Build history of the part. All positions in model axes, mm. A direction names the side the tool comes from. Round coordinates to 2 decimals unless told otherwise and drop trailing zeros. Order: outer loops, then holes, each group sorted by start corner. A loop starts at its lowest first (then second) coordinate and runs counter-clockwise, first axis right, second up. Notation, with made-up numbers: M -29,-29 L 27,-29 A18 ccw 27,-25 Z; hole C 44.5,88 d5. An arc over 180 degrees is marked long. One line per question, with ' | ' between items. Start each with the question number.
Autodesk Inventor part; units mm, degrees
ref_plane "YZ Plane" through (0, 0, 0) normal (1, 0, 0) x (0, 1, 0)
ref_plane "XZ Plane" through (0, 0, 0) normal (0, 1, 0) x (-1, 0, 0)
ref_plane "XY Plane" through (0, 0, 0) normal (0, 0, 1) x (1, 0, 0)
sketch "Boceto1" plane through (0, 0, 0) normal (0, 0, 1) x (1, 0, 0)
  line L0 (75.85, 9) -> (75.85, -9)
  line L1 (75.85, 9) -> (95.85, 9)
  line L2 (95.85, -9) -> (95.85, 9)
  line L3 (105.85, -146.9) -> (105.85, 146.9)
  line L4 (105.85, 146.9) -> (112.15, 146.9)
  line L5 (112.15, 146.9) -> (112.15, 160)
  line L6 (112.15, 160) -> (105.85, 160)
  line L7 (105.85, 160) -> (105.85, 180)
  line L8 (105.85, 180) -> (-100.9, 180)
  line L9 (-100.9, 180) -> (-100.9, 160)
  line L10 (-100.9, 160) -> (-108.4, 160)
  line L11 (-108.4, 160) -> (-108.4, 145)
  line L12 (-108.4, 145) -> (-100.9, 145)
  line L13 (-100.9, 145) -> (-100.9, 142)
  line L14 (-100.9, 142) -> (-112.15, 142)
  line L15 (-112.15, 142) -> (-112.15, -142)
  line L16 (15.85, 9) -> (15.85, -9)
  line L17 (15.85, 9) -> (35.85, 9)
  line L18 (35.85, -9) -> (35.85, 9)
  line L19 (20.45, 169.8) -> (20.45, 163.3)
  line L20 (20.45, 163.3) -> (13.95, 163.3)
  line L21 (13.95, 163.3) -> (13.95, 169.8)
  line L22 (13.95, 169.8) -> (20.45, 169.8)
  line L23 (78.15, 169.8) -> (78.15, 163.3)
  line L24 (78.15, 163.3) -> (71.65, 163.3)
  line L25 (71.65, 163.3) -> (71.65, 169.8)
  line L26 (71.65, 169.8) -> (78.15, 169.8)
  line L27 (-4.15, 163.3) -> (-4.15, 169.8)
  line L28 (-4.15, 169.8) -> (2.35, 169.8)
  line L29 (2.35, 169.8) -> (2.35, 163.3)
  line L30 (2.35, 163.3) -> (-4.15, 163.3)
  line L31 (38.55, 169.8) -> (38.55, 163.3)
  line L32 (38.55, 163.3) -> (32.05, 163.3)
  line L33 (32.05, 163.3) -> (32.05, 169.8)
  line L34 (32.05, 169.8) -> (38.55, 169.8)
  line L35 (56.65, 169.8) -> (56.65, 163.3)
  line L36 (56.65, 163.3) -> (50.15, 163.3)
  line L37 (50.15, 163.3) -> (50.15, 169.8)
  line L38 (50.15, 169.8) -> (56.65, 169.8)
  line L39 (-14.65, 175.8) -> (-14.65, 157.7)
  line L40 (-14.65, 157.7) -> (-22.65, 157.7)
  line L41 (-22.65, 157.7) -> (-22.65, 175.8)
  line L42 (-22.65, 175.8) -> (-14.65, 175.8)
  line L43 (35.85, -9) -> (35.85, 9)
  line L44 (35.85, -9) -> (15.85, -9)
  line L45 (15.85, 9) -> (15.85, -9)
  line L46 (-112.15, 142) -> (-112.15, -142)
  line L47 (-112.15, -142) -> (-100.9, -142)
  line L48 (-100.9, -142) -> (-100.9, -145)
  line L49 (-100.9, -145) -> (-108.4, -145)
  line L50 (-108.4, -145) -> (-108.4, -160)
  line L51 (-108.4, -160) -> (-100.9, -160)
  line L52 (-100.9, -160) -> (-100.9, -180)
  line L53 (-100.9, -180) -> (105.85, -180)
  line L54 (105.85, -180) -> (105.85, -160)
  line L55 (105.85, -160) -> (112.15, -160)
  line L56 (112.15, -160) -> (112.15, -146.9)
  line L57 (112.15, -146.9) -> (105.85, -146.9)
  line L58 (105.85, -146.9) -> (105.85, 146.9)
  line L59 (95.85, -9) -> (95.85, 9)
  line L60 (95.85, -9) -> (75.85, -9)
  line L61 (75.85, 9) -> (75.85, -9)
  circle A0 centre (-103.8, -156.7) radius 1.5
  line L62 (-25.85, -52.4) -> (-25.85, -57.4)
  line L63 (-25.85, -57.4) -> (-8.15, -57.4)
  arc A1 (-3.15, -62.4) -> (-8.15, -57.4) centre (-8.15, -62.4) ccw
  line L64 (-3.15, -62.4) -> (-3.15, -87.4)
  line L65 (-3.15, -87.4) -> (-2.05, -87.4)
  line L66 (-2.05, -87.4) -> (-2.05, -107.4)
  line L67 (-2.05, -107.4) -> (-3.15, -107.4)
  line L68 (-3.15, -107.4) -> (-3.15, -169.7804)
  arc A2 (-8.15, -174.7804) -> (-3.15, -169.7804) centre (-8.15, -169.7804) ccw
  line L69 (-8.15, -174.7804) -> (-67.5256, -174.7804)
  line L70 (-67.5256, -174.7804) -> (-67.5256, -57.4)
  line L71 (-67.5256, -57.4) -> (-48.05, -57.4)
  line L72 (-48.05, -57.4) -> (-48.05, -52.4)
  line L73 (-48.05, -52.4) -> (-25.85, -52.4)
  line L74 (-112.15, 0) -> (-67.15, 0)
  line L75 (-67.15, 0) -> (-67.15, -40)
  line L76 (-67.15, -40) -> (-32.15, -40)
  line L77 (-32.15, -40) -> (-32.15, 40)
  line L78 (-32.15, 40) -> (-67.15, 40)
  line L79 (-67.15, 40) -> (-67.15, 0)
  line L80 (-37.15, 35) -> (-37.15, -35)
  line L81 (-37.15, -35) -> (-62.15, -35)
  line L82 (-62.15, -35) -> (-62.15, 0)
  line L83 (-62.15, 0) -> (-62.15, 35)
  line L84 (-62.15, 35) -> (-37.15, 35)
  circle A3 centre (-37.15, 35) radius 1.5
  circle A4 centre (-37.15, -35) radius 1.5
  circle A5 centre (-62.15, -35) radius 1.5
  circle A6 centre (-62.15, 35) radius 1.5
  circle A7 centre (-37.15, -35) radius 1.6
  circle A8 centre (-37.15, 35) radius 1.6
  circle A9 centre (-62.15, 35) radius 1.6
  circle A10 centre (-62.15, -35) radius 1.6
  line L85 (75.85, 9) -> (95.85, 9)
  line L86 (15.85, 9) -> (35.85, 9)
  line L87 (20.45, 169.8) -> (20.45, 163.3)
  line L88 (20.45, 163.3) -> (13.95, 163.3)
  line L89 (13.95, 163.3) -> (13.95, 169.8)
  line L90 (13.95, 169.8) -> (20.45, 169.8)
  line L91 (78.15, 169.8) -> (78.15, 163.3)
  line L92 (78.15, 163.3) -> (71.65, 163.3)
  line L93 (71.65, 163.3) -> (71.65, 169.8)
  line L94 (71.65, 169.8) -> (78.15, 169.8)
  line L95 (-4.15, 163.3) -> (-4.15, 169.8)
  line L96 (-4.15, 169.8) -> (2.35, 169.8)
  line L97 (2.35, 169.8) -> (2.35, 163.3)
  line L98 (2.35, 163.3) -> (-4.15, 163.3)
  line L99 (38.55, 169.8) -> (38.55, 163.3)
  line L100 (38.55, 163.3) -> (32.05, 163.3)
  line L101 (32.05, 163.3) -> (32.05, 169.8)
  line L102 (32.05, 169.8) -> (38.55, 169.8)
  line L103 (56.65, 169.8) -> (56.65, 163.3)
  line L104 (56.65, 163.3) -> (50.15, 163.3)
  line L105 (50.15, 163.3) -> (50.15, 169.8)
  line L106 (50.15, 169.8) -> (56.65, 169.8)
  line L107 (-14.65, 175.8) -> (-14.65, 157.7)
  line L108 (-14.65, 157.7) -> (-22.65, 157.7)
  line L109 (-22.65, 157.7) -> (-22.65, 175.8)
  line L110 (-22.65, 175.8) -> (-14.65, 175.8)
  line L111 (-100.9, 142) -> (-112.15, 142)
  line L112 (105.85, 146.9) -> (112.15, 146.9)
  line L113 (112.15, 146.9) -> (112.15, 160)
  line L114 (112.15, 160) -> (105.85, 160)
  line L115 (105.85, 160) -> (105.85, 180)
  line L116 (105.85, 180) -> (-100.9, 180)
  line L117 (-100.9, 180) -> (-100.9, 160)
  line L118 (-100.9, 160) -> (-108.4, 160)
  line L119 (-108.4, 160) -> (-108.4, 145)
  line L120 (-108.4, 145) -> (-100.9, 145)
  line L121 (-100.9, 145) -> (-100.9, 142)
  circle A11 centre (-37.15, -35) radius 1.6
  circle A12 centre (-37.15, 35) radius 1.6
  circle A13 centre (-62.15, 35) radius 1.6
  circle A14 centre (-62.15, -35) radius 1.6
  line L122 (95.85, -9) -> (75.85, -9)
  line L123 (35.85, -9) -> (15.85, -9)
  line L124 (-25.85, -52.4) -> (-25.85, -57.4)
  line L125 (-25.85, -57.4) -> (-8.15, -57.4)
  arc A15 (-3.15, -62.4) -> (-8.15, -57.4) centre (-8.15, -62.4) ccw
  line L126 (-3.15, -62.4) -> (-3.15, -87.4)
  line L127 (-3.15, -87.4) -> (-2.05, -87.4)
  line L128 (-2.05, -87.4) -> (-2.05, -107.4)
  line L129 (-2.05, -107.4) -> (-3.15, -107.4)
  line L130 (-3.15, -107.4) -> (-3.15, -169.7804)
  arc A16 (-8.15, -174.7804) -> (-3.15, -169.7804) centre (-8.15, -169.7804) ccw
  line L131 (-8.15, -174.7804) -> (-67.5256, -174.7804)
  line L132 (-67.5256, -174.7804) -> (-67.5256, -57.4)
  line L133 (-67.5256, -57.4) -> (-48.05, -57.4)
  line L134 (-48.05, -57.4) -> (-48.05, -52.4)
  line L135 (-48.05, -52.4) -> (-25.85, -52.4)
  circle A17 centre (-103.8, -156.7) radius 1.5
  line L136 (-112.15, -142) -> (-100.9, -142)
  line L137 (-100.9, -142) -> (-100.9, -145)
  line L138 (-100.9, -145) -> (-108.4, -145)
  line L139 (-108.4, -145) -> (-108.4, -160)
  line L140 (-108.4, -160) -> (-100.9, -160)
  line L141 (-100.9, -160) -> (-100.9, -180)
  line L142 (-100.9, -180) -> (105.85, -180)
  line L143 (105.85, -180) -> (105.85, -160)
  line L144 (105.85, -160) -> (112.15, -160)
  line L145 (112.15, -160) -> (112.15, -146.9)
  line L146 (112.15, -146.9) -> (105.85, -146.9)
  dimension "d0" = 45
  dimension "d1" = 40
  dimension "d2" = 35
  dimension "d3" = 80
  dimension "d4" = 5
  dimension "d5" = 3
  dimension "d6" = 3
  dimension "d7" = 3
  dimension "d8" = 3
extrude "Extrusión1" add sketch "Boceto1" along normal blind 5 contours L79 L78 L77 L76 L75 | A3 L84 A8 L80 | L80 A8 L84 A3 | L80 A7 L81 A10 L82 L83 A9 L84 A8 | A7 L81 A4 L80 | L80 A4 L81 A7 | A9 L83 A6 L84 | L84 A6 L83 A9 | A10 L82 A5 L81 | L81 A5 L82 A10
sketch "Boceto2" plane through (0, 0, 5) normal (0, 0, 1) x (1, 0, 0)
  circle A0 centre (-37.15, 35) radius 1.5
  circle A1 centre (-62.15, -35) radius 1.5
  line L0 (-37.15, 35) -> (-62.15, 35)
  line L1 (-62.15, 35) -> (-62.15, -35)
  line L2 (-62.15, -35) -> (-37.15, -35)
  line L3 (-37.15, -35) -> (-37.15, 35)
  line L4 (-50.6099, 35) -> (-50.6099, 30)
  line L5 (-37.15, 30) -> (-62.15, 30)
  line L6 (-37.15, 25) -> (-62.15, 25)
  line L7 (-49.65, -35) -> (-49.65, -30)
  line L8 (-49.65, -25) -> (-37.15, -25)
  line L9 (-49.65, -30) -> (-37.15, -30)
  line L10 (-49.65, -30) -> (-62.15, -30)
  line L11 (-62.15, -30) -> (-37.15, -30)
  line L12 (-37.15, -30) -> (-37.15, -25)
  line L13 (-37.15, -25) -> (-62.15, -25)
  line L14 (-62.15, -25) -> (-62.15, -30)
  point P0 (0, 0)
  dimension "d11" = 5
  dimension "d12" = 5
  dimension "d13" = 5
  dimension "d14" = 5
extrude "Extrusión2" add sketch "Boceto2" along normal blind 30 contours L3 L6 L1 L5 | L3 L9 L10 L1 L13 L8
fillet "Empalme1" radius 12.5 4 edges at (-37.15, 27.5, 35) (-62.15, 27.5, 35) (-37.15, -27.5, 35) (-62.15, -27.5, 35)
fillet "Empalme2" radius 3 4 edges at (-49.65, 30, 5) (-49.65, 25, 5) (-49.65, -25, 5) (-49.65, -30, 5)
sketch "Boceto3" plane through (0, 0, 5) normal (0, 0, 1) x (1, 0, 0)
  line L0 (-62.15, -33) -> (-62.15, -22)
  line L1 (-37.15, -22) -> (-62.15, -22)
  line L2 (-37.15, -22) -> (-37.15, -33)
  line L3 (-62.15, -33) -> (-37.15, -33)
  line L4 (-62.15, 22) -> (-62.15, 33)
  line L5 (-37.15, 33) -> (-62.15, 33)
  line L6 (-37.15, 33) -> (-37.15, 22)
  line L7 (-62.15, 22) -> (-37.15, 22)
  line L8 (-32.15, 40) -> (-67.15, 40)
  line L9 (-67.15, 40) -> (-67.15, -40)
  line L10 (-67.15, -40) -> (-32.15, -40)
  line L11 (-32.15, -40) -> (-32.15, 40)
  circle A0 centre (-62.15, -35) radius 1.5
  circle A1 centre (-37.15, -35) radius 1.5
  circle A2 centre (-37.15, 35) radius 1.5
  circle A3 centre (-62.15, 35) radius 1.5
  circle A4 centre (-62.15, 35) radius 3.9
  circle A5 centre (-37.15, 35) radius 3.9
  circle A6 centre (-62.15, -35) radius 1.5
  circle A7 centre (-62.15, -35) radius 3.9
  circle A8 centre (-37.15, -35) radius 3.9
  point P0 (0, 0)
  dimension "d19" = 7.8
  dimension "d20" = 7.8
  dimension "d21" = 7.8
  dimension "d22" = 7.8
extrude "Extrusión3" cut sketch "Boceto3" along normal blind 30 contours L3 A7 L0 | L0 A7 L3 | A8 L2 L3 | L3 L2 A8 | A4 L5 L4 | L4 L5 A4 | A5 L5 L6 | L6 L5 A5
sketch "Boceto4" plane through (-49.65, 30, 22.5) normal (0, 1, 0) x (1, 0, 0)
  arc A0 (-12.5, 0) -> (12.5, 0) centre (0, 0) ccw
  point P0 (49.65, 22.5)
hole "Agujero1" at (-49.65, 30, 22.5) direction (0, -1, 0) diameter 5 depth 5 counterbore diameter 10 counterbore depth 1.6
sketch "Boceto5" plane through (-49.65, -30, 22.5) normal (0, -1, 0) x (1, 0, 0)
  arc A0 (12.5, 0) -> (-12.5, 0) centre (0, 0) ccw
  point P0 (49.65, -22.5)
hole "Agujero2" at (-49.65, -30, 22.5) direction (0, 1, 0) diameter 5 depth 5 counterbore diameter 10 counterbore depth 1.6
fillet "Empalme3" radius 5 4 edges at (-32.15, 40, 2.5) (-67.15, 40, 2.5) (-67.15, -40, 2.5) (-32.15, -40, 2.5)
properties part number "UnionBrazoPantalla"
Item 1: Cut at A-A on z = 18.5. Write the cut outline in (x, y).
Item 2: Tool access for faces 1 (the face through (-37.15, -28, 14)), 2 (the face through (-49.82, 24.14, 5.9)), 3 (the face through (-47, 30, 18)), 4 (the face through (-38.226, 31.251, 5.259)), 5 (the face through (-62.15, -27, 14)): list every direction of +Z, -Z, +X, -X, +Y, -Y with a clear straight run to the whole face (end or side of a thin tool).
Item 3: Cut at D-D on z = 12.5. Write the cut outline in (x, y).
Item 4: Cut at C-C on y = 11. Write the cut outline in (x, z).
Item 5: Two-plate mould, pull along Y, no slides. Class faces 6 (the face through (-40.909, 27.535, 31.436)), 7 (the face through (-53, -30, 18)), 8 (the face through (-49.82, -24.1, 5.86)), 9 (the face through (-61.46, 36.33, 2.46)): +Y half, -Y half, draft (parallel to the pull), parting line (faces both ways), or undercut.
Item 6: Wall check: line 1 along X through (y, z) = (35, 2.75); line 2 along Y through (x, z) = (-62.15, 1.3). Give the ranges that are in metal, low to high. Write a range as [from, to].
Item 7: Cut at B-B on z = 2. Write the cut outline in (x, y).
Item 8: Flat gauge pins, fed straight in: pin 1 (6 mm diameter, centred on x = -49.65, z = 22.5, fed in from +Y); pin 2 (2.5 mm diameter, centred on y = 27, z = 13, fed in from -X); pin 3 (6 mm diameter, centred on x = -40, y = 13.5, fed in from +Z). Where does each tip first touch, or does it go through?
Results found:
1) outline: M -62.15,-30 L -52.65,-30 L -52.65,-28.4 L -46.65,-28.4 L -46.65,-30 L -37.15,-30 L -37.15,-25 L -62.15,-25 Z; M -62.15,25 L -37.15,25 L -37.15,30 L -46.65,30 L -46.65,28.4 L -52.65,28.4 L -52.65,30 L -62.15,30 Z
2) face 1: +Z, +X, +Y, -Y | face 2: +Z, +X, -X | face 3: +Z, +X, -X, +Y | face 4: +Z, +X, +Y | face 5: +Z, -X, +Y, -Y
3) outline: M -62.15,-30 L -37.15,-30 L -37.15,-25 L -62.15,-25 Z; M -62.15,25 L -37.15,25 L -37.15,30 L -62.15,30 Z
4) outline: M -67.15,0 L -32.15,0 L -32.15,5 L -67.15,5 Z
5) face 6: draft | face 7: -Y half | face 8: undercut | face 9: undercut
6) line 1: x = [-67.15, -63.65], [-60.65, -38.65], [-35.65, -32.15] | line 2: y = [-40, -36.5], [-33.5, 33.5], [36.5, 40]
7) outline: M -67.15,-35 A5 ccw -62.15,-40 L -37.15,-40 A5 ccw -32.15,-35 L -32.15,35 A5 ccw -37.15,40 L -62.15,40 A5 ccw -67.15,35 Z; hole C -62.15,-35 d3; hole C -62.15,35 d3; hole C -37.15,-35 d3; hole C -37.15,35 d3
8) pin 1: stops at y = 28.4 | pin 2: stops at x = -62.15 | pin 3: stops at z = 5
